Drawing for the job (mm, zero at the part's lowest x, y, z). Coordinates: 2 decimals unless noted, no trailing zeros. Loops run counter-clockwise (first coordinate to the right, second up) from the corner with the lowest first, then second, coordinate; pieces in that order, holes last. Notation, with made-up numbers: (3, -4.5) -> (19, -4.5) arc R17 cw to (19, 19.5) -> close; hole circle Ø1 at (22, 33.5). An arc over 180 degrees is marked (long way). Write each question's results on one line, items separated by ' | '.
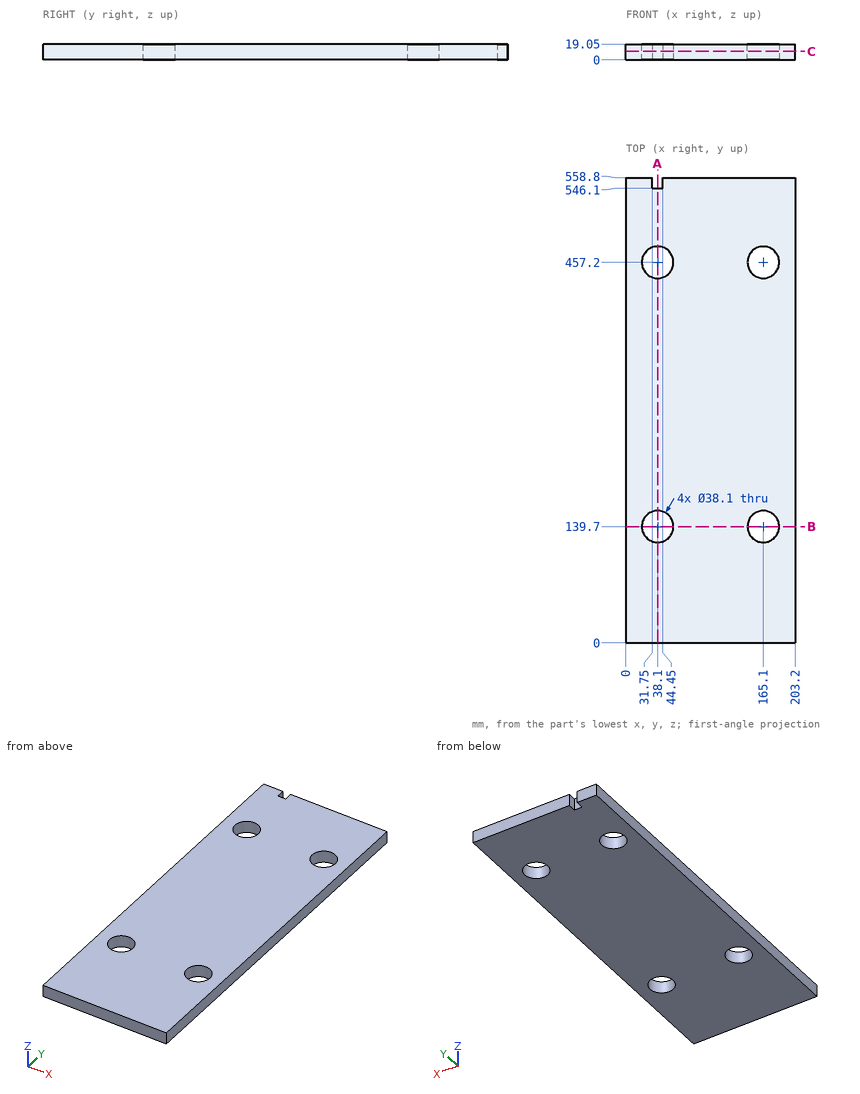
1) Slice it at C-C (z = 10.25). Write the cut outline in (x, y), then the cut area to 3 significant figures.
Outcome:
outline: (0, 0) -> (203.2, 0) -> (203.2, 558.8) -> (44.45, 558.8) -> (44.45, 546.1) -> (31.75, 546.1) -> (31.75, 558.8) -> (0, 558.8) -> close; hole circle Ø38.1 at (38.1, 139.7); hole circle Ø38.1 at (38.1, 457.2); hole circle Ø38.1 at (165.1, 139.7); hole circle Ø38.1 at (165.1, 457.2) | area: 109,000 mm^2
2) Slice it at A-A (x = 38.1). Write the cut outline in (y, z), then the cut area to 3 significant figures.
Outcome:
outline: (0, 0) -> (120.65, 0) -> (120.65, 19.05) -> (0, 19.05) -> close; (158.75, 0) -> (438.15, 0) -> (438.15, 19.05) -> (158.75, 19.05) -> close; (476.25, 0) -> (546.1, 0) -> (546.1, 19.05) -> (476.25, 19.05) -> close | area: 8,950 mm^2
3) Drill centre lines: L1, parallel to X at y = 139.7, z = 5.75; L2, parallel to Y at x = 38.1, z = 5.75; L3, parallel to Y at x = 165.1, z = 10.5. Where is each one in solid material? Low to high. Write a range as from..to.
Outcome:
L1: x = 0..19.05, 57.15..146.05, 184.15..203.2 | L2: y = 0..120.65, 158.75..438.15, 476.25..546.1 | L3: y = 0..120.65, 158.75..438.15, 476.25..558.8
4) Slice it at B-B (y = 139.7). Write the cut outline in (x, z).
Outcome:
outline: (0, 0) -> (19.05, 0) -> (19.05, 19.05) -> (0, 19.05) -> close; (57.15, 0) -> (146.05, 0) -> (146.05, 19.05) -> (57.15, 19.05) -> close; (184.15, 0) -> (203.2, 0) -> (203.2, 19.05) -> (184.15, 19.05) -> close
